Here's how the part is built. I have some questions about the finished solid (model axes, mm). Face numbers are marked on the shaded views. A direction names the side the tool comes from. Round coordinates to 2 decimals unless told otherwise and drop trailing zeros. Loops run counter-clockwise (first coordinate to the right, second up) from the corner with the lowest first, then second, coordinate; pieces in that order, holes last. Notation, with made-up numbers: (-22.75, -26) -> (20.25, -26) arc R15 cw to (20.25, -21) -> close; hole circle Ø4 at (24, 10.5). An arc over 180 degrees is marked (long way). Use CSV: the item, a comma, the result in double quotes. Start each with the question number.
from build123d import *

# Parameters (mm, degrees)
SKETCH1_W           = 20
SKETCH1_H           = 20
BOSS_EXTRUDE1_DEPTH = 1.5
SKETCH2_R           = 1.5
BOSS_EXTRUDE2_DEPTH = 1.5
SKETCH3_R           = 1
SKETCH3_R_2         = 2.5
CUT_EXTRUDE1_DEPTH  = 1.5
SKETCH4_R           = 5
BOSS_EXTRUDE3_DEPTH = 5
SKETCH5_W           = 6
SKETCH5_H           = 6
BOSS_EXTRUDE4_DEPTH = 5.5
SKETCH6_W           = 6
SKETCH6_H           = 10
BOSS_EXTRUDE5_DEPTH = 8
SKETCH7_W           = 3
SKETCH7_H           = 1.820054299
BOSS_EXTRUDE6_DEPTH = 1
SKETCH8_R           = 1.75
CUT_EXTRUDE2_DEPTH  = 0.5


with BuildPart() as part:
    # Sketch1 → Boss-Extrude1 (new body)
    with BuildSketch(Plane(origin=(0, 0, 0), x_dir=(1, 0, 0), z_dir=(0, 1, 0))):
        Rectangle(SKETCH1_W, SKETCH1_H)
    extrude(amount=BOSS_EXTRUDE1_DEPTH)

    # Sketch2 → Boss-Extrude2 (add)
    with BuildSketch(Plane(origin=(0, 1.5, 0), x_dir=(1, 0, 0), z_dir=(0, 1, 0))):
        with Locations((-10, 0)):
            Circle(SKETCH2_R)
        with Locations((10, 0)):
            Circle(SKETCH2_R)
    extrude(amount=-BOSS_EXTRUDE2_DEPTH)

    # Sketch3 → Cut-Extrude1 (cut)
    with BuildSketch(Plane(origin=(0, 1.5, 0), x_dir=(1, 0, 0), z_dir=(0, 1, 0))):
        with Locations((-10, 0)):
            Circle(SKETCH3_R)
        with Locations((10, 0)):
            Circle(SKETCH3_R)
        with Locations((0, 10)):
            Circle(SKETCH3_R_2)
        with Locations((0, -10)):
            Circle(SKETCH3_R_2)
    extrude(amount=-CUT_EXTRUDE1_DEPTH, mode=Mode.SUBTRACT)

    # Sketch4 → Boss-Extrude3 (add)
    with BuildSketch(Plane(origin=(0, 1.5, 0), x_dir=(1, 0, 0), z_dir=(0, 1, 0))):
        with Locations((-5.7, -5)):
            Circle(SKETCH4_R)
    extrude(amount=BOSS_EXTRUDE3_DEPTH)

    # Sketch5 → Boss-Extrude4 (add)
    with BuildSketch(Plane(origin=(0, 1.5, 0), x_dir=(1, 0, 0), z_dir=(0, 1, 0))):
        with Locations((-6.5, 6.5)):
            Rectangle(SKETCH5_W, SKETCH5_H)
    extrude(amount=BOSS_EXTRUDE4_DEPTH)

    # Sketch6 → Boss-Extrude5 (add)
    with BuildSketch(Plane(origin=(0, 1.5, 0), x_dir=(1, 0, 0), z_dir=(0, 1, 0))):
        with Locations((5, 0)):
            Rectangle(SKETCH6_W, SKETCH6_H)
    extrude(amount=BOSS_EXTRUDE5_DEPTH)

    # Sketch7 → Boss-Extrude6 (add)
    with BuildSketch(Plane(origin=(0, 1.5, 0), x_dir=(1, 0, 0), z_dir=(0, 1, 0))):
        with Locations((-0.5, 4.292954161)):
            Rectangle(SKETCH7_W, SKETCH7_H)
    extrude(amount=BOSS_EXTRUDE6_DEPTH)

    # Sketch8 → Cut-Extrude2 (cut)
    with BuildSketch(Plane(origin=(0, 7, 0), x_dir=(1, 0, 0), z_dir=(0, 1, 0))):
        with Locations((-6.5, 6.5)):
            Circle(SKETCH8_R)
    extrude(amount=-CUT_EXTRUDE2_DEPTH, mode=Mode.SUBTRACT)


solid = part.part
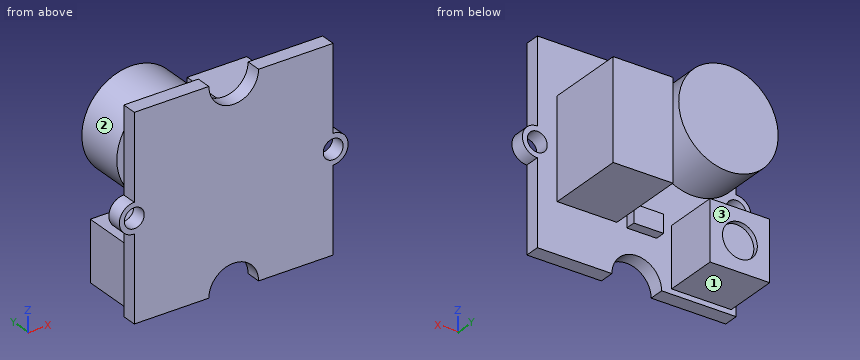
Q1. For the marked faces 1, 2 and 3, which set-ups out of +Z, -Z, +X, -X, +Y, -Y let a thin tool reach every point of the face, with its end or its side?
Q2. Will these pins go through, and if not, where does the flat tip stop? pin 1 Ø1.5 at (x, y) = (-3, 5) entering from +Z; pin 2 Ø4 at (y, z) = (6.5, 1) entering from -X; pin 3 Ø3 at (x, y) = (-7.5, 4.5) entering from -Z.
Q3. I want a section at D-D, the plane z = -5.5. List the corners of the cut face in (x, y) for me, then the cut area to 3 significant figures.
Q4. I want a section at C-C, the plane y = 0.75. List the corners of the cut face in (x, z) for me.
Q5. I want a section at B-B, the plane x = 0. List the corners of the cut face in (y, z) for me.
Q6. I need wall thicknesses on line 1 along X through (y, z) = (0.9, 0); line 2 along Z through (x, y) = (-6.5, 6.6); line 3 along Z through (x, y) = (7.5, 4.5). Which ranges of each line are inside material? Lowest first, please.
Q7. I want a section at A-A, the plane y = 3. List the corners of the cut face in (x, z) for me, then the cut area to 3 significant figures.
Values found:
1,face 1,"-Z, +X, -X, +Y"
1,face 2,"+Y"
1,face 3,"+Z, -Z, -X, +Y"
2,pin 1,"z = 9.6"
2,pin 2,"x = -10.28"
2,pin 3,"z = -9.5"
3,outline,"(-10, 0) -> (10, 0) -> (10, 1.5) -> (-3.5, 1.5) -> (-3.5, 7) -> (-5.06, 7) -> (-5.06, 6.5) -> (-7.94, 6.5) -> (-7.94, 7) -> (-9.5, 7) -> (-9.5, 1.5) -> (-10, 1.5) -> close"
3,area,"61.6 mm2"
4,outline,"(-10, -10) -> (-2.5, -10) arc R2.5 cw to (2.5, -10) -> (10, -10) -> (10, -1.5) arc R1.5 ccw to (10, 1.5) -> (10, 10) -> (2.5, 10) arc R2.5 cw to (-2.5, 10) -> (-10, 10) -> (-10, 1.5) arc R1.5 ccw to (-10, -1.5) -> close; hole circle Ø2 at (-10, 0); hole circle Ø2 at (10, 0)"
5,outline,"(0, -7.5) -> (1.5, -7.5) -> (1.5, -5.2) -> (2.5, -5.2) -> (2.5, -3.38) -> (1.5, -3.38) -> (1.5, 7.5) -> (0, 7.5) -> close"
6,line 1,"-11.5 to -11, -9 to 9, 11 to 11.5"
6,line 2,"-9.5 to -8.25, -4.75 to -3.5"
6,line 3,"-5 to 5"
7,outline,"circle Ø10 at (-5.7, 5); (-9.5, -9.5) -> (-3.5, -9.5) -> (-3.5, -3.5) -> (-9.5, -3.5) -> close; (2, -5) -> (8, -5) -> (8, 5) -> (2, 5) -> close"
7,area,"175 mm2"
